For this review, take the finished solid that the model builds, in its own axes (mm). Give positions to 0.01 mm unless a question says otherwise; leave off trailing zeros. Write each loop counter-clockwise with the first axis right and the second up, starting at its lowest first coordinate (ties: lowest second). Pieces come first, ordered by that corner, then holes. Notation, with made-up numbers: (53, -38.75) -> (91, -38.75) arc R16 ccw to (91, -32.75) -> close; hole circle Ø8 at (-24, 11). An arc over 180 degrees is marked (long way). Answer as CSV lines item,"result".
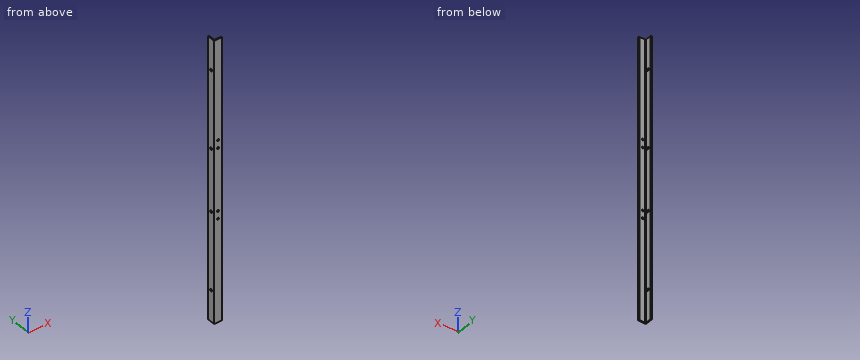
```python
from build123d import *

# Parameters (mm, degrees)
BOSS_EXTRUDE1_DEPTH                 = 914.4
F_13_16_0_8125_DIAMETER_HOLE1_D     = 12.7
F_13_16_0_8125_DIAMETER_HOLE1_DEPTH = 6.35
F_5_8_0_625_DIAMETER_HOLE1_D        = 15.875
F_5_8_0_625_DIAMETER_HOLE1_DEPTH    = 6.35
SKETCH7_R                           = 6.35
CUT_EXTRUDE1_DEPTH                  = 7.35


with BuildPart() as part:
    # Sketch1 → Boss-Extrude1 (new body, symmetric)
    with BuildSketch(Plane.XY):
        with BuildLine():
            Line((0, 0), (0, 50.8))
            Line((0, 50.8), (1.59258, 50.8))
            ThreePointArc((1.59258, 50.8), (4.956583943, 49.406583943), (6.35, 46.04258))
            Line((6.35, 46.04258), (6.35, 11.1125))
            ThreePointArc((6.35, 11.1125), (7.744903955, 7.744903955), (11.1125, 6.35))
            Line((11.1125, 6.35), (46.04258, 6.35))
            ThreePointArc((46.04258, 6.35), (49.406583943, 4.956583943), (50.8, 1.59258))
            Line((50.8, 1.59258), (50.8, 0))
            Line((50.8, 0), (0, 0))
        make_face()
    extrude(amount=BOSS_EXTRUDE1_DEPTH, both=True)

    # 13/16 (0.8125) Diameter Hole1
    with Locations(Plane.XZ):
        with Locations((25.4, -195.834), (25.4, 210.566)):
            Hole(F_13_16_0_8125_DIAMETER_HOLE1_D / 2, depth=F_13_16_0_8125_DIAMETER_HOLE1_DEPTH)

    # 5/8 (0.625) Diameter Hole1
    with Locations(Plane.ZY):
        with Locations((-711.2, 25.4), (-203.2, 25.4), (203.2, 25.4), (711.2, 25.4)):
            Hole(F_5_8_0_625_DIAMETER_HOLE1_D / 2, depth=F_5_8_0_625_DIAMETER_HOLE1_DEPTH)

    # Sketch7 → Cut-Extrude1 (cut, through all)
    with BuildSketch(Plane(origin=(0, 6.35, 0), x_dir=(1, 0, 0), z_dir=(0, 1, 0))):
        with Locations((25.4, 246.634)):
            Circle(SKETCH7_R)
        with Locations((25.4, -261.366)):
            Circle(SKETCH7_R)
    extrude(amount=-CUT_EXTRUDE1_DEPTH, mode=Mode.SUBTRACT)


solid = part.part
```
Q1. Add section A-A (y = 25.4). Write out the cut boundary in (x, z), plus the area to 3 significant figures.
Answer block:
outline,"(0, -914.4) -> (6.35, -914.4) -> (6.35, -719.14) -> (0, -719.14) -> close; (0, -703.26) -> (6.35, -703.26) -> (6.35, -211.14) -> (0, -211.14) -> close; (0, -195.26) -> (6.35, -195.26) -> (6.35, 195.26) -> (0, 195.26) -> close; (0, 211.14) -> (6.35, 211.14) -> (6.35, 703.26) -> (0, 703.26) -> close; (0, 719.14) -> (6.35, 719.14) -> (6.35, 914.4) -> (0, 914.4) -> close"
area,"11,200 mm2"
Q2. Clearance check with flat-ended pins moving along their axes: pin 1 (10.5 mm diameter, centred on x = 27.5, z = -256, fed in from +Y); pin 2 (2 mm diameter, centred on y = 32.5, z = 348, fed in from +X); pin 3 (9.5 mm diameter, centred on y = 25.4, z = -711.2, fed in from +X); pin 4 (12 mm diameter, centred on x = 9.5, z = 391.5, fed in from +Y). State where each tip first meets the part, or that it passes through.
Answer block:
pin 1,"stops at y = 6.35"
pin 2,"stops at x = 6.35"
pin 3,"passes through"
pin 4,"stops at y = 50.4"
Q3. To check wall thickness, follow probe 1 along Z at (x, y) = (25, 3); probe 2 along Z at (x, y) = (2, 25); probe 3 along X at (y, z) = (41, 625). State the ranges of each line that lie inside material, in increasing order. Write a range as [from, to].
Answer block:
probe 1,"z = [-914.4, -252.97], [-240.3, -202.17], [-189.5, 204.23], [216.9, 255.03], [267.7, 914.4]"
probe 2,"z = [-914.4, -719.13], [-703.27, -211.13], [-195.27, 195.27], [211.13, 703.27], [719.13, 914.4]"
probe 3,"x = [0, 6.35]"
